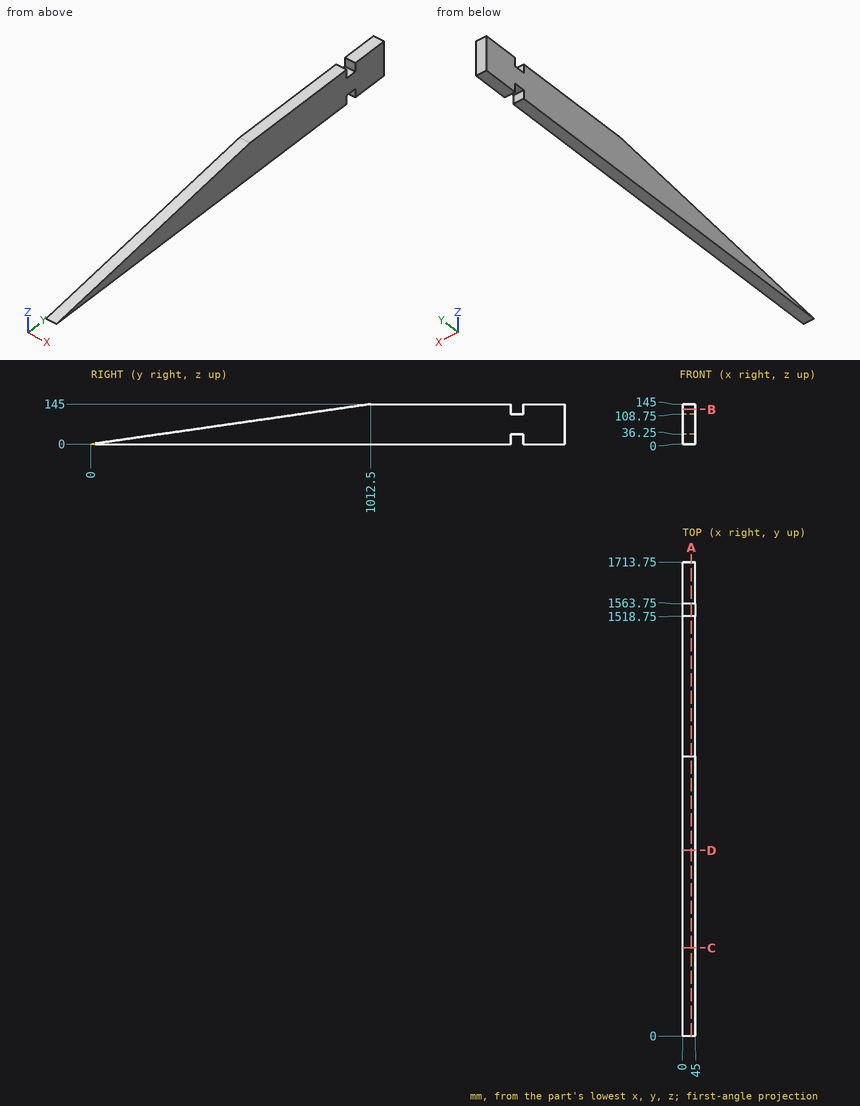
Input: dimensioned drawing with shaded views. Units: mm. Origin: part minimum x, y, z. Coordinates: 2 decimals unless noted, no trailing zeros. Loops run counter-clockwise (first coordinate to the right, second up) from the corner with the lowest first, then second, coordinate; pieces in that order, holes last. Notation, with made-up numbers: M 60,55 L 100,55 A23 cw 100,72 Z; hole C 6,19 d4. An arc over 180 degrees is marked long. Use a Markdown table: item, result. Add a question column.
Q1. Material intervals for L1, parallel to Z at x = 24, y = 1556.5; L2, parallel to Z at x = 10.5, y = 314, sorted ascending.
Q2. First-contact query: pin 1 (13.5 mm diameter, centred on x = 16.5, y = 1542.5, fed in from -Z). Flat tip, straight axial feed; report the tip coordinate or a pass-through.
Q3. Section query C-C, the plane y = 318.5. Return loops of the section in (x, z).
Q4. Section query D-D, the plane y = 671.5. Return loops of the section in (x, z).
Q5. Section query A-A, the plane x = 31. Return loops of the section in (y, z).
Q6. Section query B-B, the plane z = 125.5. Return loops of the section in (x, y).
Result:
| question | item | result |
|---|---|---|
| 1 | L1 | z = 36.25 to 108.75 |
| 1 | L2 | z = 0 to 44.97 |
| 2 | pin 1 | stops at z = 36.25 |
| 3 | outline | M 0,0 L 45,0 L 45,45.61 L 0,45.61 Z |
| 4 | outline | M 0,0 L 45,0 L 45,96.17 L 0,96.17 Z |
| 5 | outline | M 0,0 L 1518.75,0 L 1518.75,36.25 L 1563.75,36.25 L 1563.75,0 L 1713.75,0 L 1713.75,145 L 1563.75,145 L 1563.75,108.75 L 1518.75,108.75 L 1518.75,145 L 1012.5,145 Z |
| 6 | outline | M 0,876.34 L 45,876.34 L 45,1518.75 L 0,1518.75 Z; M 0,1563.75 L 45,1563.75 L 45,1713.75 L 0,1713.75 Z |
